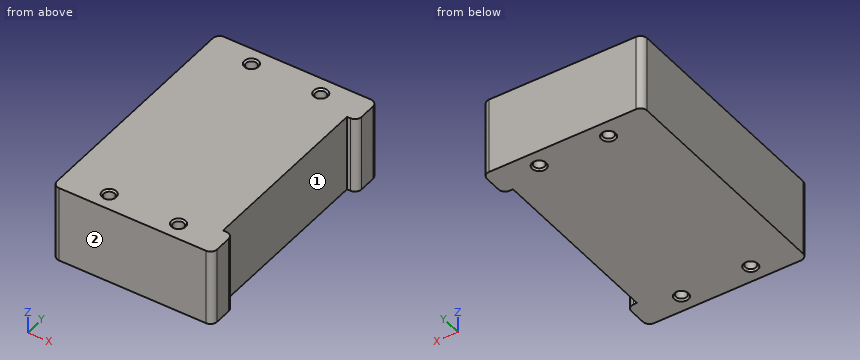
Autodesk Inventor part; units mm, degrees
ref_plane "Work Plane1" through (0, 0, 0) normal (0, 0, 1) x (1, 0, 0)
ref_plane "YZ Plane" through (0, 0, 0) normal (1, 0, 0) x (0, 1, 0)
ref_plane "XZ Plane" through (0, 0, 0) normal (0, 1, 0) x (-1, 0, 0)
ref_plane "Work Plane1" through (0, 0, 0) normal (0, 0, 1) x (1, 0, 0)
sketch "Sketch1" plane through (0, 0, 0) normal (0, 0, 1) x (1, 0, 0)
  line L0 (-42.2638, -6.6778) -> (-4.2638, -6.6778)
  line L1 (-44.2638, -77.1778) -> (-44.2638, -8.6778)
  line L2 (-4.2638, -79.1778) -> (-42.2638, -79.1778)
  line L3 (-2.2638, -8.6778) -> (-2.2638, -77.1778)
  circle A0 centre (-23.2638, -42.9278) radius 12.6
  circle A1 centre (-7.2638, -42.9278) radius 2
  circle A2 centre (-23.2638, -58.9278) radius 2
  circle A3 centre (-11.9501, -54.2415) radius 1.5
  circle A4 centre (-34.5775, -54.2415) radius 1.5
  circle A5 centre (-11.9501, -31.6141) radius 1.5
  circle A6 centre (-23.2638, -26.9278) radius 2
  circle A7 centre (-34.5775, -31.6141) radius 1.5
  circle A8 centre (-39.2638, -42.9278) radius 2
  arc A9 (-38.6638, -72.0778) -> (-38.6638, -76.2778) centre (-38.6638, -74.1778) ccw
  line L4 (-7.8638, -72.0778) -> (-38.6638, -72.0778)
  arc A10 (-7.8638, -76.2778) -> (-7.8638, -72.0778) centre (-7.8638, -74.1778) ccw
  line L5 (-38.6638, -76.2778) -> (-7.8638, -76.2778)
  arc A11 (-7.8638, -13.7778) -> (-7.8638, -9.5778) centre (-7.8638, -11.6778) ccw
  line L6 (-38.6638, -13.7778) -> (-7.8638, -13.7778)
  arc A12 (-38.6638, -9.5778) -> (-38.6638, -13.7778) centre (-38.6638, -11.6778) ccw
  line L7 (-7.8638, -9.5778) -> (-38.6638, -9.5778)
  line L8 (30.6247, -21.3479) -> (-25.1038, -35.8635)
  arc A13 (-25.1038, -35.8635) -> (-25.1038, -49.9921) centre (-23.2638, -42.9278) ccw
  line L9 (-25.1038, -49.9921) -> (30.6247, -64.5078)
  arc A14 (30.6247, -64.5078) -> (30.6247, -21.3479) centre (36.2457, -42.9278) ccw
  arc A15 (-24.9022, -36.6377) -> (-24.9022, -49.2179) centre (-23.2638, -42.9278) ccw
  line L10 (30.8264, -22.122) -> (-24.9022, -36.6377)
  arc A16 (30.8264, -63.7336) -> (30.8264, -22.122) centre (36.2457, -42.9278) ccw
  line L11 (-24.9022, -49.2179) -> (30.8264, -63.7336)
  line L12 (-44.2638, -15.6778) -> (-2.2638, -15.6778)
  line L13 (-2.2638, -70.1778) -> (-44.2638, -70.1778)
  line L14 (-35.2638, -68.1778) -> (-35.2638, -17.6778)
  line L15 (-47.2638, -8.6778) -> (-47.2638, -77.1778)
  line L16 (-45.2638, -6.6778) -> (-4.2638, -6.6778)
  line L17 (-45.2638, -79.1778) -> (-4.2638, -79.1778)
  arc A17 (-45.2638, -6.6778) -> (-47.2638, -8.6778) centre (-45.2638, -8.6778) ccw
  arc A18 (-47.2638, -77.1778) -> (-45.2638, -79.1778) centre (-45.2638, -77.1778) ccw
  arc A19 (-33.2638, -15.6778) -> (-35.2638, -17.6778) centre (-33.2638, -17.6778) ccw
  arc A20 (-35.2638, -68.1778) -> (-33.2638, -70.1778) centre (-33.2638, -68.1778) ccw
  line L18 (0.7362, -72.1778) -> (0.7362, -77.1778)
  line L19 (0.7362, -8.6778) -> (0.7362, -13.6778)
  line L20 (-2.2638, -15.6778) -> (-1.2638, -15.6778)
  line L21 (-4.2638, -6.6778) -> (-1.2638, -6.6778)
  line L22 (-2.2638, -70.1778) -> (-1.2638, -70.1778)
  line L23 (-4.2638, -79.1778) -> (-1.2638, -79.1778)
  arc A21 (0.7362, -8.6778) -> (-1.2638, -6.6778) centre (-1.2638, -8.6778) ccw
  arc A22 (-1.2638, -15.6778) -> (0.7362, -13.6778) centre (-1.2638, -13.6778) ccw
  arc A23 (0.7362, -72.1778) -> (-1.2638, -70.1778) centre (-1.2638, -72.1778) ccw
  arc A24 (-1.2638, -79.1778) -> (0.7362, -77.1778) centre (-1.2638, -77.1778) ccw
  line L24 (-44.2638, -70.1778) -> (-44.2638, -15.6778)
  arc A25 (-2.2638, -8.6778) -> (-4.2638, -6.6778) centre (-4.2638, -8.6778) ccw
  arc A26 (-42.2638, -6.6778) -> (-44.2638, -8.6778) centre (-42.2638, -8.6778) ccw
  arc A27 (-44.2638, -77.1778) -> (-42.2638, -79.1778) centre (-42.2638, -77.1778) ccw
  arc A28 (-4.2638, -79.1778) -> (-2.2638, -77.1778) centre (-4.2638, -77.1778) ccw
  point P0 (0, 0)
  point P1 (-35.2638, -15.6778)
  point P2 (-35.2638, -70.1778)
  point P3 (-12.8638, -11.6778)
  point P4 (-33.6638, -11.6778)
  point P5 (-33.6638, -74.1778)
  point P6 (-12.8638, -74.1778)
  point P7 (-35.2638, -55.5753)
  point P8 (-35.2638, -52.9077)
  point P9 (-35.2638, -46.7697)
  point P10 (-35.2638, -39.0859)
  point P11 (-35.2638, -32.9479)
  point P12 (-35.2638, -30.2803)
  point P13 (-47.2638, -6.6778)
  point P14 (-47.2638, -79.1778)
  point P15 (0.7362, -70.1778)
  point P16 (0.7362, -79.1778)
  point P17 (0.7362, -6.6778)
  point P18 (0.7362, -15.6778)
  point P19 (-42.2638, -6.6778)
  dimension "d0" = 9
  dimension "d1" = 9
  dimension "d2" = 9
  dimension "d3" = 5
  dimension "d4" = 5
  dimension "d5" = 5
  dimension "d6" = 5
  dimension "d9" = 3
  dimension "d12" = 3
  dimension "d13" = 3
extrude "Extrusion1" add sketch "Sketch1" along normal blind 23 contours A26 L1 A27 L17 A18 L15 A17 L16 | L0 A25 L3 L12 L1 A26 | L21 A21 L19 A22 L20 L3 A25 | L12 A19 L14 A7 A0 A4 A20 L13 L1 | L3 L8 A5 A0 L14 A7 A19 L12 | L13 L3 A28 L2 A27 L1 | L3 L10 A0 L8 A5 | A20 L14 A4 A0 L9 A3 L3 L13 | L3 L11 A0 L10 | L8 A5 | A5 L8 | L22 A23 L18 A24 L23 A28 L3 | L14 A7 | A7 L14 | L3 L9 A3 A0 L11 | L10 A15 L11 A0 L9 A13 L8 | A0 L11 A15 L10 | L14 A4 | A4 L14 | L8 A13 L9 A0 L14 | L9 A3 | A3 L9 | L14 A0 | A1 | A2 | A6 | A8 | L4 A10 L5 A9 | L6 A12 L7 A11
sketch "Sketch2" plane through (0, 0, 23) normal (0, 0, 1) x (1, 0, 0)
  arc A0 (-1.2638, -15.6778) -> (0.7362, -13.6778) centre (-1.2638, -13.6778) ccw
  line L0 (0.7362, -13.6778) -> (0.7362, -8.6778)
  arc A1 (0.7362, -8.6778) -> (-1.2638, -6.6778) centre (-1.2638, -8.6778) ccw
  arc A2 (-45.2638, -6.6778) -> (-47.2638, -8.6778) centre (-45.2638, -8.6778) ccw
  line L1 (-47.2638, -8.6778) -> (-47.2638, -77.1778)
  arc A3 (-47.2638, -77.1778) -> (-45.2638, -79.1778) centre (-45.2638, -77.1778) ccw
  arc A4 (-1.2638, -79.1778) -> (0.7362, -77.1778) centre (-1.2638, -77.1778) ccw
  line L2 (0.7362, -77.1778) -> (0.7362, -72.1778)
  arc A5 (0.7362, -72.1778) -> (-1.2638, -70.1778) centre (-1.2638, -72.1778) ccw
  line L3 (-1.2638, -70.1778) -> (-2.2638, -70.1778)
  line L4 (-2.2638, -15.6778) -> (-1.2638, -15.6778)
  line L5 (-2.2638, -70.1778) -> (-2.2638, -15.6778)
  line L6 (-1.2638, -6.6778) -> (-45.2638, -6.6778)
  line L7 (-45.2638, -79.1778) -> (-1.2638, -79.1778)
  point P0 (0, 0)
  point P1 (-12.8638, -11.6778)
  point P2 (-33.6638, -11.6778)
  point P3 (-33.6638, -74.1778)
  point P4 (-12.8638, -74.1778)
hole "Hole1" at (-12.8638, -11.6778, 23) at (-33.6638, -11.6778, 23) at (-33.6638, -74.1778, 23) at (-12.8638, -74.1778, 23) direction (0, 0, -1) diameter 3.242 end through all
chamfer "Chamfer1" distance 0.5 angle 45 8 edges at (-33.6638, -72.5568, 23) (-12.8638, -72.5568, 23) (-33.6638, -10.0568, 23) (-12.8638, -10.0568, 23) (-33.6638, -72.5568, 0) (-12.8638, -72.5568, 0) (-33.6638, -10.0568, 0) (-12.8638, -10.0568, 0)
equation "\"d1\" = d2"
equation "\"d2\" = d0"
equation "\"d12\" = d9"
equation "\"d13\" = d12"
properties part number "hoefijzer"
Geometry check sheet. Reference: the model listing, model coordinates, mm. Face numbers are marked on the shaded views. A direction names the side the tool comes from. Coordinates: 2 decimals unless noted, no trailing zeros. Order: outer loops, then holes, each group sorted by start corner. A loop starts at its lowest first (then second) coordinate and runs counter-clockwise, first axis right, second up.
Q1. Thickness scan on probe 1 along Y at (x, z) = (-13, 17.5); probe 2 along Y at (x, z) = (-11.5, 4.5); probe 3 along X at (y, z) = (-39, 21.5). Record the ranges inside material, lowest first.
Reply:
probe 1: y = -79.18 to -75.79, -72.56 to -13.29, -10.06 to -6.68
probe 2: y = -79.18 to -75.05, -73.3 to -12.55, -10.8 to -6.68
probe 3: x = -47.26 to -2.26
Q2. Depth check by flat-ended pin: pin 1 Ø3 at (x, y) = (-12.86, -74.18) entering from +Z; pin 2 Ø7 at (y, z) = (-50.5, 9.5) entering from +X; pin 3 Ø6 at (x, y) = (-11.5, -14) entering from -Z; pin 4 Ø4 at (x, y) = (-33.66, -74.18) entering from -Z. Enter the tip coordinate at first touch or a pass-through.
Reply:
pin 1: passes through
pin 2: stops at x = -2.26
pin 3: stops at z = 0
pin 4: stops at z = 0.12
Q3. Sectioned sample at B-B on y = -21. Record the cut outline in (x, z).
Reply:
outline: (-47.26, 0) - (-2.26, 0) - (-2.26, 23) - (-47.26, 23) - close
Q4. Tool access check on the marked faces 1 and 2. Record the directions out of +Z, -Z, +X, -X, +Y, -Y that give a thin tool (end or side, any length) a straight path to the whole face; none if there is none.
Reply:
face 1: +Z, -Z, +X
face 2: +Z, -Z, +X, -X, -Y
Q5. Sectioned sample at A-A on z = 2.5. Record the cut outline in (x, y).
Reply:
outline: (-47.26, -77.18) arc R2 ccw to (-45.26, -79.18) - (-1.26, -79.18) arc R2 ccw to (0.74, -77.18) - (0.74, -72.18) arc R2 ccw to (-1.26, -70.18) - (-2.26, -70.18) - (-2.26, -15.68) - (-1.26, -15.68) arc R2 ccw to (0.74, -13.68) - (0.74, -8.68) arc R2 ccw to (-1.26, -6.68) - (-45.26, -6.68) arc R2 ccw to (-47.26, -8.68) - close; hole circle Ø3.24 at (-33.66, -74.18); hole circle Ø3.24 at (-33.66, -11.68); hole circle Ø3.24 at (-12.86, -74.18); hole circle Ø3.24 at (-12.86, -11.68)
